Verification items for the finished model (mm, model axes). A direction names the side the tool comes from. Coordinates: 2 decimals unless noted, no trailing zeros. Write each loop counter-clockwise with the first axis right and the second up, starting at its lowest first coordinate (ties: lowest second). Pieces come first, ordered by that corner, then holes. Notation, with made-up numbers: (-8.5, -25) -> (15.5, -25) arc R9 ccw to (15.5, -8) -> close; hole circle Ø2 at (45, 10). An arc over 180 degrees is marked (long way). Use CSV: the item, a comma, the result in double quotes.
```python
from build123d import *
from OCP.BRepFilletAPI import BRepFilletAPI_MakeChamfer

# Parameters (mm, degrees)
EXTRUDE_1_DEPTH = 10
CHAMFER_4_SIZE  = 4
CHAMFER_4_SIZE2 = 1.455880937
EXTRUDE_2_DEPTH = 3


with BuildPart() as part:
    # 草图1 → 凸台-拉伸1 (new body)
    with BuildSketch(Plane.XY):
        Polygon((-12.5, 7.5), (-14.508805155, 0.156246539), (-12.5, -7.5), (12.5, -7.5), (14.508805155, 0.156246539), (12.5, 7.5), align=None)
    extrude(amount=EXTRUDE_1_DEPTH)

    # 倒角4: one chamfer whose edges measure the first distance from different faces: ONE call of the kernel's chamfer builder (chamfer() names one face for all edges)
    chamfer_4_edges_1 = [part.edges().sort_by_distance(p)[0] for p in [
        (-13.504402578, 3.82812327, 10),
    ]]
    chamfer_4_side_1 = [part.faces().sort_by_distance(p)[0] for p in [
        (-13.504402578, 3.82812327, 5),
    ]]
    chamfer_4_edges_2 = [part.edges().sort_by_distance(p)[0] for p in [
        (-13.504402578, -3.67187673, 10),
    ]]
    chamfer_4_side_2 = [part.faces().sort_by_distance(p)[0] for p in [
        (-13.504402578, -3.67187673, 5),
    ]]
    chamfer_4_edges_3 = [part.edges().sort_by_distance(p)[0] for p in [
        (0, -7.5, 10),
    ]]
    chamfer_4_side_3 = [part.faces().sort_by_distance(p)[0] for p in [
        (0, -7.5, 5),
    ]]
    chamfer_4_edges_4 = [part.edges().sort_by_distance(p)[0] for p in [
        (13.504402578, -3.67187673, 10),
    ]]
    chamfer_4_side_4 = [part.faces().sort_by_distance(p)[0] for p in [
        (13.504402578, -3.67187673, 5),
    ]]
    chamfer_4_edges_5 = [part.edges().sort_by_distance(p)[0] for p in [
        (13.504402578, 3.82812327, 10),
    ]]
    chamfer_4_side_5 = [part.faces().sort_by_distance(p)[0] for p in [
        (13.504402578, 3.82812327, 5),
    ]]
    chamfer_4_edges_6 = [part.edges().sort_by_distance(p)[0] for p in [
        (0, 7.5, 10),
    ]]
    chamfer_4_side_6 = [part.faces().sort_by_distance(p)[0] for p in [
        (0, 7.5, 5),
    ]]
    chamfer_4 = BRepFilletAPI_MakeChamfer(part.part.solid().wrapped)
    for e in chamfer_4_edges_1:
        chamfer_4.Add(CHAMFER_4_SIZE, CHAMFER_4_SIZE2, e.wrapped, chamfer_4_side_1[0].wrapped)  # the first distance lies on this face
    for e in chamfer_4_edges_2:
        chamfer_4.Add(CHAMFER_4_SIZE, CHAMFER_4_SIZE2, e.wrapped, chamfer_4_side_2[0].wrapped)  # the first distance lies on this face
    for e in chamfer_4_edges_3:
        chamfer_4.Add(CHAMFER_4_SIZE, CHAMFER_4_SIZE2, e.wrapped, chamfer_4_side_3[0].wrapped)  # the first distance lies on this face
    for e in chamfer_4_edges_4:
        chamfer_4.Add(CHAMFER_4_SIZE, CHAMFER_4_SIZE2, e.wrapped, chamfer_4_side_4[0].wrapped)  # the first distance lies on this face
    for e in chamfer_4_edges_5:
        chamfer_4.Add(CHAMFER_4_SIZE, CHAMFER_4_SIZE2, e.wrapped, chamfer_4_side_5[0].wrapped)  # the first distance lies on this face
    for e in chamfer_4_edges_6:
        chamfer_4.Add(CHAMFER_4_SIZE, CHAMFER_4_SIZE2, e.wrapped, chamfer_4_side_6[0].wrapped)  # the first distance lies on this face
    add(Compound.cast(chamfer_4.Shape()), mode=Mode.REPLACE)

    # 草图4 → 凸台-拉伸2 (add)
    with BuildSketch(Plane.XY.offset(10)):
        Polygon((-0.842329886, 4.204878172), (-0.997111855, 3.082708897), (-0.875425349, 3.0960765), (-0.88342019, 3.010417485), (-0.615021943, 2.973869638), (-0.997111855, 1.451293683), (-1.286540896, 1.419499093), (-1.593044591, 0.977341926), (-2.107271415, 0.920852672), (1.898363481, 0.85858655), (1.373153369, 0.990387846), (1.096764689, 1.369234669), (0.769770761, 1.451293683), (0.417287548, 2.992143562), (0.684395911, 3.053246992), (0.684395911, 3.120908441), (0.790079324, 3.120908441), (0.637139108, 4.204878172), (0.353273229, 4.243532249), (0.31846389, 3.870575043), (0.095475844, 3.870575043), (0.054505452, 4.243532249), (-0.248639641, 4.243532249), (-0.28344898, 3.870575043), (-0.496098331, 3.847214918), (-0.539634898, 4.243532249), align=None)
        Polygon((-1.210689891, 0.977341926), (-0.783853716, 0.977341926), (-0.697469796, 1.321570013), (-0.266044311, 1.451293683), (-0.806066899, 1.451293683), (-0.991003184, 1.395685902), align=None, mode=Mode.SUBTRACT)
        Polygon((-0.806066899, 1.521254444), (-0.364830167, 1.521254444), (-0.29903642, 1.713574629), (-0.43352874, 1.784201139), (-0.517866614, 1.828489836), (-0.635596744, 1.693330399), (-0.417971271, 1.693330399), (-0.585448533, 1.617414536), (-0.774567684, 1.617414536), align=None, mode=Mode.SUBTRACT)
    extrude(amount=EXTRUDE_2_DEPTH)


solid = part.part
```
1) Gauge pin test, flat ends, axial feed: pin 1 (2 mm diameter, centred on x = 6.5, z = 9, fed in from -Y); pin 2 (0.5 mm diameter, centred on x = -0.5, z = 12, fed in from +Y); pin 3 (1 mm diameter, centred on y = -5, z = 5.5, fed in from -X); pin 4 (3.5 mm diameter, centred on x = -1.5, y = 2.5, fed in from +Z). Record the tip position at first contact, or that the pin passes through.
Return value:
pin 1,"y = -6.77"
pin 2,"y = 4.24"
pin 3,"x = -13.29"
pin 4,"z = 13"
2) Cross-section at A-A (z = 1.5). Record the boundary of the cut face in (x, y).
Return value:
outline,"(-14.51, 0.16) -> (-12.5, -7.5) -> (12.5, -7.5) -> (14.51, 0.16) -> (12.5, 7.5) -> (-12.5, 7.5) -> close"
3) Cross-section at C-C (z = 11). Give the number of separate pieces and of enclosed holes in the cut face, plus the area to 3 significant figures.
Return value:
separate pieces,"1"
enclosed holes,"2"
area,"5.24 mm2"
4) Mould release check, pull along Y, two halves, no side actions. Record for faces 1 (the flat face through (-0.803, 2.223, 11.479)), 2 (the flat face through (13.518, 3.777, 2.958)), 3 (the flat face through (-12.804, -3.431, 8.028)): released by +Y, released by -Y, zero draft, split by the parting line, or undercut.
Return value:
face 1,"undercut"
face 2,"released by +Y"
face 3,"released by -Y"
5) Cross-section at B-B (x = 2.75). Record the boundary of the cut face in (y, z), plus the area to 3 significant figures.
Return value:
outline,"(-7.5, 0) -> (7.5, 0) -> (7.5, 6) -> (6.04, 10) -> (-6.04, 10) -> (-7.5, 6) -> close"
area,"144 mm2"
6) Scan lines: L1, parallel to Z at x = 4.25, y = -1; L2, parallel to X at y = 3.25, z = 7.75; L3, parallel to X at y = 1.25, z = 10.75. Record each from-to range of solid material in increasing order.
Return value:
L1,"0 to 10"
L2,"-13 to 13"
L3,"-1.4 to -1.07, -0.72 to 1.18"
7) Cross-section at D-D (y = 2.5). Record the boundary of the cut face in (x, z), plus the area to 3 significant figures.
Return value:
outline,"(-13.87, 0) -> (13.87, 0) -> (13.87, 6) -> (12.36, 10) -> (0.53, 10) -> (0.53, 13) -> (-0.73, 13) -> (-0.73, 10) -> (-12.36, 10) -> (-13.87, 6) -> close"
area,"275 mm2"
8) Set-up check for faces 4 (the flat face through (-0.92, 3.65, 11.48)), 5 (the flat face through (0.715, 3.655, 11.479)), 6 (the flat face through (-0.17, -6.76, 8.03)): record each of +Z, -Z, +X, -X, +Y, -Y from which the full face is reachable in a straight line by a thin tool's end or side.
Return value:
face 4,"+Z, -X, +Y"
face 5,"+Z, +X, +Y"
face 6,"+Z, +X, -X, -Y"
